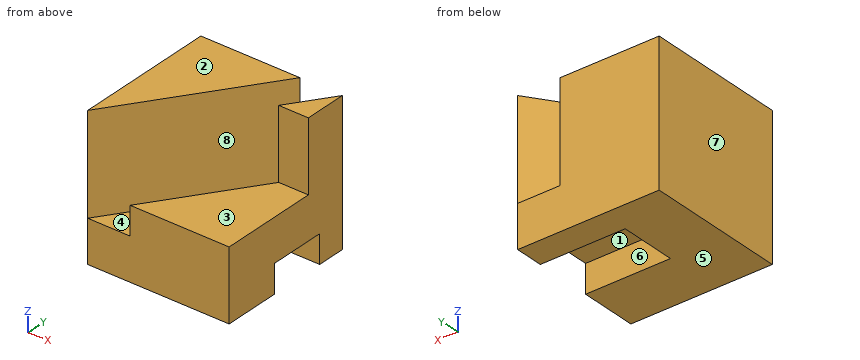
```python
from build123d import *

# Parameters (mm, degrees)
F0_W     = 50
F0_H     = 50
F1_DEPTH = 50
F3_DEPTH = 35
F4_W     = 20
F4_H     = 10
F5_DEPTH = 30
F7_DEPTH = 25


with BuildPart() as f1:
    # F0 (on Top) → F1 (new body)
    with BuildSketch(Plane.XY):
        with Locations((25, 25)):
            Rectangle(F0_W, F0_H)
    extrude(amount=F1_DEPTH)

    # F2 (on face) → F3 (cut)
    with BuildSketch(Plane.XY.offset(50)):
        Polygon((15, 0), (50, 50), (35, 50), (0, 0), align=None)
    extrude(amount=-F3_DEPTH, mode=Mode.SUBTRACT)

    # F4 (on face) → F5 (cut)
    with BuildSketch(Plane.YZ.offset(50)):
        with Locations((30, 5)):
            Rectangle(F4_W, F4_H)
    extrude(amount=-F5_DEPTH, mode=Mode.SUBTRACT)

    # F6 (on face) → F7 (cut)
    with BuildSketch(Plane.XY.offset(50)):
        Polygon((50, 35), (39.5, 35), (15, 0), (50, 0), align=None)
    extrude(amount=-F7_DEPTH, mode=Mode.SUBTRACT)


solid = f1.part
```
Read the model definition and answer for the solid it produces. Units are mm, in the model's axes. Face numbers are marked on the shaded views. A direction names the side the tool comes from. Coordinates: 2 decimals unless noted, no trailing zeros. Order: outer loops, then holes, each group sorted by start corner. A loop starts at its lowest first (then second) coordinate and runs counter-clockwise, first axis right, second up. Notation, with made-up numbers: (18.25, 61.5) - (50.25, 61.5) arc R26 ccw to (50.25, 100.5) - close; hole circle Ø6 at (7, 10.25). An arc over 180 degrees is marked (long way). Answer as a JSON object with one key per item and string values. Group by question number.
Item 1: Consider probe 1 along Y at (x, z) = (33, 8.5); probe 2 along Z at (x, y) = (34.5, 39.5); probe 3 along X at (y, z) = (43.5, 33.5). Determine where each line is inside the solid, lowest interval first. Write a range as from..to.
Item 2: Section D-D (z = 4) is taken. Give the vertices of the cut face in (x, y), plus the area to 3 significant figures.
Item 3: Section C-C (x = 7) is taken. Give the vertices of the cut face in (y, z), plus the area to 3 significant figures.
Item 4: Flat-ended cylindrical pins translate along their axes: P1, Ø10, axis at x = 42.5, y = 27, coming from the -Z side; P2, Ø11.5, axis at x = 46, z = 43, coming from the -Y side; P3, Ø11, axis at y = 32, z = 3, coming from the +X side. Find the tip coordinate at first contact, or state that the pin passes through.
Item 5: The mould has two halves that part along X. Classify the marked faces 6, 7 and 8: +X half, -X half, draft (parallel to the pull), parting line (faces both ways), or undercut.
Item 6: Section B-B (y = 39) is taken. Give the vertices of the cut face in (x, z).
Item 7: A tool of negligible diameter and unlimited length cuts with its end or side. For the marked faces 1, 2, 3, 4 and 5, from which of +Z, -Z, +X, -X, +Y, -Y can it reach the whole face along a straight path? Write none if from no direction.
Item 8: Section A-A (z = 17) is taken. Give the vertices of the cut face in (x, y), plus the area to 3 significant figures.
Results are:
{
 "1": {"probe 1": "y = 0..20, 40..50", "probe 2": "z = 10..15", "probe 3": "x = 0..30.45, 45.45..50"},
 "2": {"outline": "(0, 0) - (50, 0) - (50, 20) - (20, 20) - (20, 40) - (50, 40) - (50, 50) - (0, 50) - close", "area": "1,900 mm^2"},
 "3": {"outline": "(0, 0) - (50, 0) - (50, 50) - (10, 50) - (10, 15) - (0, 15) - close", "area": "2,150 mm^2"},
 "4": {"P1": "stops at z = 10", "P2": "stops at y = 35", "P3": "stops at x = 20"},
 "5": {"face 6": "draft", "face 7": "-X half", "face 8": "undercut"},
 "6": {"outline": "(0, 0) - (20, 0) - (20, 10) - (50, 10) - (50, 50) - (42.3, 50) - (42.3, 15) - (27.3, 15) - (27.3, 50) - (0, 50) - close"},
 "7": {"face 1": "-Z, +X", "face 2": "+Z, +X, -X, +Y, -Y", "face 3": "+Z, +X, -Y", "face 4": "+Z", "face 5": "-Z, +X, -X, +Y, -Y"},
 "8": {"outline": "(0, 0) - (35, 50) - (0, 50) - close; (15, 0) - (50, 0) - (50, 50) - close", "area": "1,750 mm^2"}
}
